Autodesk Fusion 360 part; units mm, degrees
sketch "Sketch1" plane through (0, 0, 0) normal (0, 0, 1) x (1, 0, 0)
  line L0 (70, 70) -> (-70, 70)
  line L1 (-70, 70) -> (-70, -70)
  line L2 (-70, -70) -> (70, -70)
  line L3 (70, -70) -> (70, 70)
  line L4 (70, 70) -> (-70, -70) construction
  line L5 (-70, 70) -> (70, -70) construction
  line L6 (0, 70) -> (0, 105)
  line L7 (0, 105) -> (0, 112.5)
  circle A0 centre (0, 105) radius 7.5
  line L8 (-70, 70) -> (-3.9815, 111.3559)
  line L9 (3.9815, 111.3559) -> (70, 70)
  circle A1 centre (0, 105) radius 2.5
  dimension "d1" = 140
  dimension "d2" = 140
  dimension "d3" = 35
  dimension "d4" = 7.5
  dimension "d5" = 5
extrude "Extrude1" add sketch "Sketch1" along normal blind 5 contours L0 L1 L2 L3 | L0 L6 A0 L9 | L0 L6 A0 L8 | L6 L7 A0 A1 | L6 L7 A0 A1
sketch "Sketch2" plane through (0, 0, 5) normal (0, 0, 1) x (-1, 0, 0)
  circle A0 centre (0, -105) radius 2.5
  line L0 (70, -70) -> (70, 70)
  line L1 (70, 70) -> (-70, 70)
  line L2 (-70, 70) -> (-70, -70)
  line L3 (-70, -70) -> (-3.9815, -111.3559)
  arc A1 (-3.9815, -111.3559) -> (3.9815, -111.3559) centre (0, -105) ccw
  line L4 (3.9815, -111.3559) -> (70, -70)
  line L5 (70, -70) -> (70, 70)
  line L6 (70, 70) -> (-70, 70)
  line L7 (-70, 70) -> (-70, -70)
  line L8 (68, 68) -> (-68, 68)
  line L9 (-68, 68) -> (-68, -68)
  line L10 (68, -68) -> (68, 68)
  line L11 (68, -68) -> (68, -70)
  line L12 (-68, -68) -> (-68, -70)
  line L13 (-70, -70) -> (-68, -70)
  line L14 (68, -70) -> (70, -70)
  dimension "d8" = 2
  dimension "d9" = 2
  dimension "d10" = 2
extrude "Extrude2" add sketch "Sketch2" along normal blind 35 contours L0 L1 L2 L5 L6 L7 L8 L9 L10 L11 L12 L13 L14
sketch "Sketch3" plane through (0, 0, 5) normal (0, 0, 1) x (-1, 0, 0)
  line L0 (-68, -70) -> (-70, -70)
  line L1 (-70, -70) -> (-3.9815, -111.3559)
  arc A0 (-3.9815, -111.3559) -> (3.9815, -111.3559) centre (0, -105) ccw
  line L2 (3.9815, -111.3559) -> (70, -70)
  line L3 (70, -70) -> (68, -70)
  line L4 (68, -70) -> (68, 68)
  line L5 (68, 68) -> (-68, 68)
  line L6 (-68, 68) -> (-68, -70)
  circle A1 centre (0, -105) radius 2.5
  circle A2 centre (-38, 38) radius 1.5
  line L7 (-38, 38) -> (10, 38)
  circle A3 centre (10, 38) radius 1.5
  circle A4 centre (-14, 38) radius 20
  line L8 (-14, 58) -> (-14, 18)
  line L9 (-13, 58) -> (-15, 58)
  line L10 (-15, 58) -> (-15, 18)
  line L11 (-15, 18) -> (-13, 18)
  line L12 (-13, 18) -> (-13, 58)
  line L13 (-13, 58) -> (-15, 18) construction
  line L14 (-15, 58) -> (-13, 18) construction
  line L15 (6, 37) -> (-34, 37)
  line L16 (-34, 37) -> (-34, 39)
  line L17 (-34, 39) -> (6, 39)
  line L18 (6, 39) -> (6, 37)
  line L19 (6, 37) -> (-34, 39) construction
  line L20 (-34, 37) -> (6, 39) construction
  line L21 (-14, 38) -> (-23.1711, 38)
  line L22 (-14, 38) -> (-23.1711, 38)
  line L23 (-24, 20.6795) -> (-24, 55.3205)
  line L24 (-24.1711, 55.2206) -> (-24.1711, 20.7794)
  line L25 (-22.1711, 19.7453) -> (-22.1711, 56.2547)
  line L26 (-22.9946, 55.8633) -> (-23.3458, 20.3179) construction
  line L27 (-23.3458, 55.6821) -> (-22.9946, 20.1367) construction
  line L28 (-14, 38) -> (-4, 38)
  line L29 (-5, 55.8606) -> (-5, 20.1394)
  line L30 (-3, 21.2967) -> (-3, 54.7033)
  line L31 (-3.3211, 54.9104) -> (-4.7111, 20.288) construction
  line L32 (-4.7111, 55.712) -> (-3.3211, 21.0896) construction
  line L33 (-14, 38) -> (-14, 48)
  line L34 (3.8606, 47) -> (-31.8606, 47)
  line L35 (-30.7033, 49) -> (2.7033, 49)
  line L36 (3.8606, 47) -> (-30.7443, 48.9375) construction
  line L37 (-31.8606, 47) -> (2.7443, 48.9375) construction
  line L38 (-14, 38) -> (-14, 28)
  line L39 (3.8606, 29) -> (-31.8606, 29)
  line L40 (-30.7033, 27) -> (2.7033, 27)
  line L41 (3.7436, 28.7715) -> (-30.8756, 27.2663) construction
  line L42 (-31.7436, 28.7715) -> (2.8756, 27.2663) construction
  point P0 (-14, 38)
  point P1 (-14, 38)
  point P2 (-23.1711, 38)
  point P3 (-4, 38)
  point P4 (-14, 48)
  point P5 (-14, 28)
  dimension "d14" = 3
  dimension "d15" = 30
  dimension "d16" = 30
  dimension "d17" = 48
  dimension "d18" = 3
  dimension "d19" = 40
  dimension "d22" = 40
  dimension "d23" = 2
  dimension "d24" = 40
  dimension "d25" = 2
  dimension "d27" = 10
  dimension "d30" = 10
  dimension "d32" = 10
extrude "Extrude4" cut sketch "Sketch3" against normal blind 10 contours A2 | A3 | A4 L17 L24 L34 | A4 L15 L24 L39 | A4 L24 L35 | A4 L24 L40 | L10 L15 L25 L39 | L10 L17 L25 L34 | A4 L10 L25 L40 | A4 L10 L25 L35 | L12 L15 L29 L39 | L12 L17 L29 L34 | A4 L12 L29 L40 | A4 L15 L30 L39 | A4 L12 L29 L35 | A4 L17 L30 L34 | A4 L30 L40 | A4 L30 L35
extrude "Extrude3" [suppressed]
The model under review builds one solid part; all positions refer to its coordinate system, in mm. A direction names the side the tool comes from. Coordinates: 2 decimals unless noted, no trailing zeros. Write each loop counter-clockwise with the first axis right and the second up, starting at its lowest first coordinate (ties: lowest second). Pieces come first, ordered by that corner, then holes. Notation, with made-up numbers: (1.5, 85.5) -> (13.5, 85.5) arc R12 cw to (13.5, 106.5) -> close; hole circle Ø11 at (58.25, -3.5). An arc over 180 degrees is marked (long way). One line per item, written item: value. Start each with the question number.
Q1. The part is to be moulded in two halves that separate along X. For faces 1 (the face through (-1, -70, 20)), 2 (the face through (3, -52, 3)), say which applies: +X half, -X half, draft (parallel to the pull), parting line (faces both ways), or undercut.
Q2. Add section C-C, the plane z = 15.5. Give the boundary of the cut face in (x, y).
Q3. To check wall thickness, follow probe 1 along X at (y, z) = (-38, 3.8); probe 2 along X at (y, z) = (-45.5, 32); probe 3 along Z at (x, y) = (25, 78). State the ranges of each line that lie inside material, in increasing order.
Q4. Add section A-A, the plane x = 19.5. Give the boundary of the cut face in (y, z), then the cut area to 3 significant figures.
Q5. Clearance check with flat-ended pins moving along their axes: P1, Ø1, axis at x = 39.5, y = 47, coming from the +Z side; P2, Ø4, axis at x = 18.5, z = 2.5, coming from the +Y side; P3, Ø1.5, axis at x = 8.5, z = 1.5, coming from the +Y side. State where each tip first meets the part, or that it passes through.
Q6. For faces 3 (the face through (-1, 2, 0)), 4 (the face through (9, -49, 3)), list the 3-axis set-ups (+Z, -Z, +X, -X, +Y, -Y) from which the entire face can be reached by the end or side of a thin tool; tool diameter is ignored.
Q7. Add section B-B, the plane y = 105. Give the boundary of the cut face in (x, z).
Q8. Add section D-D, the plane y = 60. Give the boundary of the cut face in (x, z), then the cut area to 3 significant figures.
Response:
1. face 1: draft
1. face 2: undercut
2. outline: (-70, -70) -> (70, -70) -> (70, 70) -> (68, 70) -> (68, -68) -> (-68, -68) -> (-68, 70) -> (-70, 70) -> close
3. probe 1: -70 to -11.5, -8.5 to 36.5, 39.5 to 70
3. probe 2: -70 to -68, 68 to 70
3. probe 3: 0 to 5
4. outline: (-70, 0) -> (-57.23, 0) -> (-57.23, 5) -> (-68, 5) -> (-68, 40) -> (-70, 40) -> close; (-49, 0) -> (-47, 0) -> (-47, 5) -> (-49, 5) -> close; (-39, 0) -> (-37, 0) -> (-37, 5) -> (-39, 5) -> close; (-29, 0) -> (-27, 0) -> (-27, 5) -> (-29, 5) -> close; (-18.77, 0) -> (101.63, 0) -> (101.63, 5) -> (-18.77, 5) -> close
4. area: 766 mm²
5. P1: z = 5
5. P2: y = 103.51
5. P3: y = 109
6. face 3: -Z, +X, -X, +Y, -Y
6. face 4: +Z, -Z
7. outline: (-14.13, 0) -> (-2.5, 0) -> (-2.5, 5) -> (-14.13, 5) -> close; (2.5, 0) -> (14.13, 0) -> (14.13, 5) -> (2.5, 5) -> close
8. outline: (-70, 0) -> (70, 0) -> (70, 40) -> (68, 40) -> (68, 5) -> (-68, 5) -> (-68, 40) -> (-70, 40) -> close
8. area: 840 mm²
